Build history of the part. All positions in model axes, mm. Round coordinates to 2 decimals unless told otherwise and drop trailing zeros. Write each loop counter-clockwise with the first axis right and the second up, starting at its lowest first coordinate (ties: lowest second). Pieces come first, ordered by that corner, then holes. Notation, with made-up numbers: M 75,-9.5 L 132,-9.5 A8 cw 132,-1.5 Z; hole C 65,62 d5. An arc over 180 degrees is marked long. Write item = value, one per line. Start each with the question number.
Q1. Probe L1, parallel to X at y = -62, z = 2.55 (3 decimals); L2, parallel to X at y = 101.5, z = 2; L3, parallel to Y at x = 27, z = 1.8. List the from-to ranges inside material, lowest first.
Q2. Band-saw the part on B-B on y = 14.5. Write the cut outline in (x, z).
Q3. Band-saw the part on A-A on y = -129. Write the cut outline in (x, z), plus the area to 3 significant figures.
Q4. Band-saw the part on C-C on z = 1.65. State how many separate pieces and enclosed holes the cut face has, plus the area to 3 significant figures.
Q5. Drop flat-ended pins along their axis: P1, Ø0.9, axis at x = 71.5, z = 2, coming from the -Y side; P2, Ø4.5, axis at x = -82.55, y = -120.65, coming from the +Z side. Give the stop position or say it passes through.
```python
from build123d import *

# Parameters (mm, degrees)
F0_R     = 2.50063
F0_R_2   = 1.5875
F0_R_3   = 3.175
F0_W     = 30.40126
F0_H     = 38.1
F0_W_2   = 6.35
F0_H_2   = 6.35
F0_W_3   = 5
F0_H_3   = 164.866201
F0_W_4   = 54.61
F0_H_4   = 19.05
F1_DEPTH = 3


with BuildPart() as f1:
    # F0 (on Top) → F1 (new body)
    with BuildSketch(Plane.XY):
        with BuildLine():
            Line((44.45, 89.174706), (88.9, 89.174706))
            Line((88.9, 89.174706), (88.9, 139.974706))
            Line((88.9, 139.974706), (-88.9, 139.974706))
            Line((-88.9, 139.974706), (-88.9, 89.174706))
            Line((-88.9, 89.174706), (-44.45, 89.174706))
            Line((-44.45, 89.174706), (-88.9, 76.2))
            Line((-88.9, 76.2), (-88.9, -88.632697))
            Line((-88.9, -88.632697), (-44.45, -107.682697))
            Line((-44.45, -107.682697), (-88.9, -107.682697))
            Line((-88.9, -107.682697), (-88.9, -158.482697))
            Line((-88.9, -158.482697), (-6.35, -158.482697))
            Line((-6.35, -158.482697), (-6.35, -174.357697))
            ThreePointArc((-6.35, -174.357697), (-4.490128, -178.847825), (0, -180.707697))
            ThreePointArc((0, -180.707697), (4.490128, -178.847825), (6.35, -174.357697))
            Line((6.35, -174.357697), (6.35, -158.482697))
            Line((6.35, -158.482697), (88.9, -158.482697))
            Line((88.9, -158.482697), (88.9, -107.682697))
            Line((88.9, -107.682697), (44.45, -107.682697))
            Line((44.45, -107.682697), (88.9, -88.632697))
            Line((88.9, -88.632697), (88.9, 66.949706))
            Line((88.9, 66.949706), (88.9, 76.2))
            Line((88.9, 76.2), (44.45, 89.174706))
        make_face()
        with Locations((-82.55, -146.05)):
            Circle(F0_R, mode=Mode.SUBTRACT)
        with Locations((-82.55, -120.65)):
            Circle(F0_R, mode=Mode.SUBTRACT)
        with Locations((-36.805, -152.403702)):
            Circle(F0_R, mode=Mode.SUBTRACT)
        with Locations((-21.55063, -145.782697)):
            Circle(F0_R, mode=Mode.SUBTRACT)
        with Locations((-36.805, -107.682697)):
            Circle(F0_R, mode=Mode.SUBTRACT)
        with Locations((-21.55063, -120.382697)):
            Circle(F0_R, mode=Mode.SUBTRACT)
        with Locations((-12.7, -109.266495)):
            Circle(F0_R, mode=Mode.SUBTRACT)
        with Locations((-61.595, -82.020102)):
            Circle(F0_R_2, mode=Mode.SUBTRACT)
        with Locations((-60.325, -33.760102)):
            Circle(F0_R_2, mode=Mode.SUBTRACT)
        with Locations((-9.525, -76.940102)):
            Circle(F0_R_2, mode=Mode.SUBTRACT)
        with Locations((-9.525, -49.000102)):
            Circle(F0_R_2, mode=Mode.SUBTRACT)
        with Locations((0, -174.357697)):
            Circle(F0_R_3, mode=Mode.SUBTRACT)
        with Locations((21.55063, -145.782697)):
            Circle(F0_R, mode=Mode.SUBTRACT)
        with Locations((36.805, -152.403702)):
            Circle(F0_R, mode=Mode.SUBTRACT)
        with Locations((0, -133.078995)):
            Rectangle(F0_W, F0_H, mode=Mode.SUBTRACT)
        with Locations((21.55063, -120.382697)):
            Circle(F0_R, mode=Mode.SUBTRACT)
        with Locations((12.7, -109.266495)):
            Circle(F0_R, mode=Mode.SUBTRACT)
        with Locations((36.805, -107.682697)):
            Circle(F0_R, mode=Mode.SUBTRACT)
        with Locations((82.55, -145.782697)):
            Circle(F0_R, mode=Mode.SUBTRACT)
        with Locations((82.55, -120.382697)):
            Circle(F0_R, mode=Mode.SUBTRACT)
        with Locations((19.05, -64.816495)):
            Rectangle(F0_W_2, F0_H_2, mode=Mode.SUBTRACT)
        with Locations((0, -21.833394)):
            Rectangle(F0_W_3, F0_H_3, mode=Mode.SUBTRACT)
        with Locations((69.85, -64.816495)):
            Rectangle(F0_W_2, F0_H_2, mode=Mode.SUBTRACT)
        with Locations((-36.805, 0)):
            Circle(F0_R, mode=Mode.SUBTRACT)
        with Locations((-82.55, 101.874706)):
            Circle(F0_R, mode=Mode.SUBTRACT)
        with Locations((-82.55, 127.274706)):
            Circle(F0_R, mode=Mode.SUBTRACT)
        with BuildLine():
            ThreePointArc((-41.671875, 64.644375), (-39.6875, 66.62875), (-37.703125, 64.644375))
            Line((-37.703125, 64.644375), (-37.703125, 62.612375))
            ThreePointArc((-37.703125, 62.612375), (-39.6875, 60.628), (-41.671875, 62.612375))
            Line((-41.671875, 62.612375), (-41.671875, 64.644375))
        make_face(mode=Mode.SUBTRACT)
        with Locations((-36.805, 89.174706)):
            Circle(F0_R, mode=Mode.SUBTRACT)
        with BuildLine():
            Line((-22.621875, 62.612375), (-22.621875, 64.644375))
            ThreePointArc((-22.621875, 64.644375), (-20.6375, 66.62875), (-18.653125, 64.644375))
            Line((-18.653125, 64.644375), (-18.653125, 62.612375))
            ThreePointArc((-18.653125, 62.612375), (-20.6375, 60.628), (-22.621875, 62.612375))
        make_face(mode=Mode.SUBTRACT)
        with Locations((-12.7, 90.762206)):
            Circle(F0_R, mode=Mode.SUBTRACT)
        with Locations((-36.805, 133.353702)):
            Circle(F0_R, mode=Mode.SUBTRACT)
        with Locations((-21.55063, 101.603702)):
            Circle(F0_R, mode=Mode.SUBTRACT)
        with Locations((-21.55063, 127.003702)):
            Circle(F0_R, mode=Mode.SUBTRACT)
        with Locations((36.805, 0)):
            Circle(F0_R, mode=Mode.SUBTRACT)
        with Locations((19.05, 43.133505)):
            Rectangle(F0_W_2, F0_H_2, mode=Mode.SUBTRACT)
        with Locations((69.85, 43.133505)):
            Rectangle(F0_W_2, F0_H_2, mode=Mode.SUBTRACT)
        with Locations((0, 76.474706)):
            Rectangle(F0_W_4, F0_H_4, mode=Mode.SUBTRACT)
        with Locations((12.7, 90.762206)):
            Circle(F0_R, mode=Mode.SUBTRACT)
        with Locations((36.805, 89.174706)):
            Circle(F0_R, mode=Mode.SUBTRACT)
        with Locations((0, 114.574706)):
            Rectangle(F0_W, F0_H, mode=Mode.SUBTRACT)
        with Locations((21.55063, 101.603702)):
            Circle(F0_R, mode=Mode.SUBTRACT)
        with Locations((21.55063, 127.003702)):
            Circle(F0_R, mode=Mode.SUBTRACT)
        with Locations((36.805, 133.353702)):
            Circle(F0_R, mode=Mode.SUBTRACT)
        with Locations((82.55, 101.874706)):
            Circle(F0_R, mode=Mode.SUBTRACT)
        with Locations((82.55, 127.274706)):
            Circle(F0_R, mode=Mode.SUBTRACT)
    extrude(amount=F1_DEPTH)


solid = f1.part
```
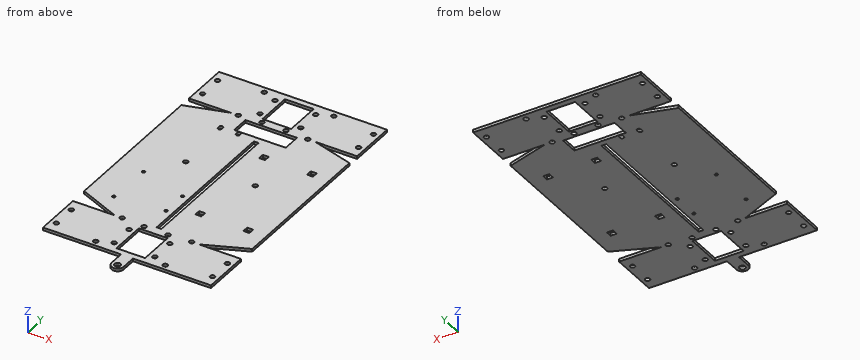
Conclusion:
q1.L1 = -88.9 to -2.5, 2.5 to 15.875, 22.225 to 66.675, 73.025 to 88.9
q1.L2 = -88.9 to -85.02, -80.08 to -24.05, -19.05 to -15.2, 15.2 to 19.05, 24.05 to 80.08, 85.02 to 88.9
q1.L3 = -158.48 to 66.95, 86 to 139.97
q2.outline = M -88.9,0 L -2.5,0 L -2.5,3 L -88.9,3 Z; M 2.5,0 L 88.9,0 L 88.9,3 L 2.5,3 Z
q3.outline = M -88.9,0 L -15.2,0 L -15.2,3 L -88.9,3 Z; M 15.2,0 L 88.9,0 L 88.9,3 L 15.2,3 Z
q3.area = 442 mm^2
q4.separate_pieces = 1
q4.enclosed_holes = 45
q4.area = 46,900 mm^2
q5.P1 = -158.48
q5.P2 = through
